Verification items for this drawing (mm, ordinates from the low corner). A direction names the side the tool comes from. Give positions to 0.01 mm unless a question says otherwise; leave off trailing zeros. Write each loop counter-clockwise with the first axis right and the second up, starting at its lowest first coordinate (ties: lowest second). Pieces come first, ordered by that corner, then holes. Notation, with made-up numbers: (24, 32.25) -> (40, 32.25) arc R19 cw to (40, 54.25) -> close; hole circle Ø10 at (53, 14). An arc over 180 degrees is marked (long way). Use one line per item in the form item = value. Start each with the question number.
(1) Section check A-A, the plane x = 16.5. Record the cut outline in (y, z).
(2) Scan lines: L1, parallel to Y at x = 17.5, z = 9.5; L2, parallel to X at y = 31.5, z = 3.75; L3, parallel to X at y = 53.5, z = 11.5. Record each from-to range of solid material in increasing order.
(3) Section check C-C, the plane y = 22.5. Record the cut outline in (x, z), plus the area to 3 significant figures.
(4) Release check for a two-part mould opening along X. For the marked faces 1, 2 and 3 record: pulls with the +X half, pulls with the -X half, needs draft (parallel to the pull), parting line crosses it, or undercut.
(5) Section check D-D, the plane x = 6. Record the cut outline in (y, z), plus the area to 3 significant figures.
(6) Section check B-B, the plane z = 1.75. Record the cut outline in (x, y).
(7) Depth check by flat-ended pin: pin 1 Ø2 at (y, z) = (54.5, 13.5) entering from +X; pin 2 Ø5.5 at (x, z) = (6, 11.5) entering from +Y; pin 3 Ø2.5 at (x, z) = (4, 10.5) entering from -Y. Enter the tip coordinate at first touch or a pass-through.
(8) Set-up check for the marked faces 4, 5 and 6: record each of +Z, -Z, +X, -X, +Y, -Y from which the full face is reachable in a straight line by a thin tool's end or side.
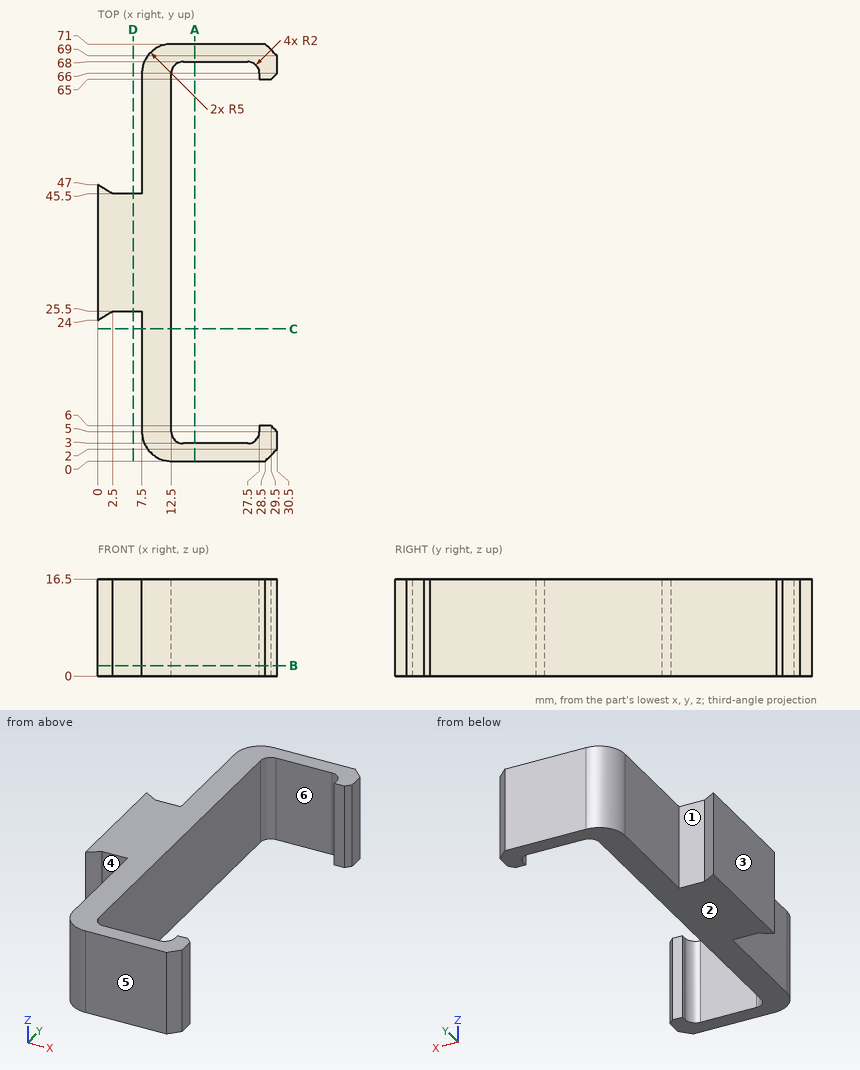
Completed:
q1.outline = (0, 0) -> (3, 0) -> (3, 16.5) -> (0, 16.5) -> close; (68, 0) -> (71, 0) -> (71, 16.5) -> (68, 16.5) -> close
q2.L1 = 0 to 3, 68 to 71
q2.L2 = 0 to 12.5
q2.L3 = 7.5 to 12.5
q3.outline = (7.5, 0) -> (12.5, 0) -> (12.5, 16.5) -> (7.5, 16.5) -> close
q3.area = 82.5 mm²
q4.face_1 = undercut
q4.face_2 = needs draft
q4.face_3 = pulls with the -X half
q5.outline = (25.5, 0) -> (45.5, 0) -> (45.5, 16.5) -> (25.5, 16.5) -> close
q5.area = 330 mm²
q6.outline = (0, 24) -> (2.5, 25.5) -> (7.5, 25.5) -> (7.5, 5) arc R5 ccw to (12.5, 0) -> (28.5, 0) -> (30.5, 2) -> (30.5, 5) -> (29.5, 6) -> (27.5, 6) -> (27.5, 5) arc R2 cw to (25.5, 3) -> (14.5, 3) arc R2 cw to (12.5, 5) -> (12.5, 66) arc R2 cw to (14.5, 68) -> (25.5, 68) arc R2 cw to (27.5, 66) -> (27.5, 65) -> (29.5, 65) -> (30.5, 66) -> (30.5, 69) -> (28.5, 71) -> (12.5, 71) arc R5 ccw to (7.5, 66) -> (7.5, 45.5) -> (2.5, 45.5) -> (0, 47) -> close
q7.pin_1 = 12.5
q7.pin_2 = 69.31
q7.pin_3 = 25.5
q8.face_4 = +Z, -Z, -Y
q8.face_5 = +Z, -Z, +X, -X, -Y
q8.face_6 = +Z, -Z
